Part print with two shaded views. Sizes in mm from the minimum x, y, z corner. A direction names the side the tool comes from. Round coordinates to 2 decimals unless told otherwise and drop trailing zeros. Order: outer loops, then holes, each group sorted by start corner. A loop starts at its lowest first (then second) coordinate and runs counter-clockwise, first axis right, second up. Notation, with made-up numbers: (38.25, 41.25) -> (82.25, 41.25) arc R18 cw to (82.25, 72.25) -> close; hole circle Ø11 at (74.5, 58). An arc over 180 degrees is marked (long way). Put each result on its own line as item: value. Start each with the question number.
Q1. Cut at A-A, the plane x = 62. List the corners of the cut face in (y, z) (3 decimals).
Q2. Cut at C-C, the plane z = 83.5. List the corners of the cut face in (x, y) (3 decimals).
Q3. Cut at D-D, the plane y = 91.5. List the corners of the cut face in (x, z) (3 decimals).
Q4. Probe L1, parallel to Z at x = 78, y = 137 (3 decimals); L2, parallel to X at y = 112, z = 59 (3 decimals); L3, parallel to Z at x = 91.5, y = 128. List the from-to ranges inside material, lowest first.
Q5. 3-axis set-ups, long thin cutter, end or side, ignore diameter. For the marked faces 5, 6, 7 and 8: which of +Z, -Z, +X, -X, +Y, -Y reach the whole face in a straight line?
Q6. Cut at B-B, the plane y = 141.5. List the corners of the cut face in (x, z) (3 decimals).
Q7. Flat gauge pins, fed straight in: P1, Ø4, axis at y = 65.5, z = 87.5, coming from the +X side; P2, Ø15, axis at y = 26, z = 79, coming from the +X side; P3, Ø15, axis at y = 82.5, z = 89, coming from the -X side; P4, Ø1.5, axis at x = 47.5, y = 135, coming from the -Z side. Where does each tip first touch, or does it go through?
Q8. Pull direction Z, two halves, no side cores. Call the marked faces 1, 2, 3 and 4: released by +Z, released by -Z, zero draft, split by the parting line, or undercut.
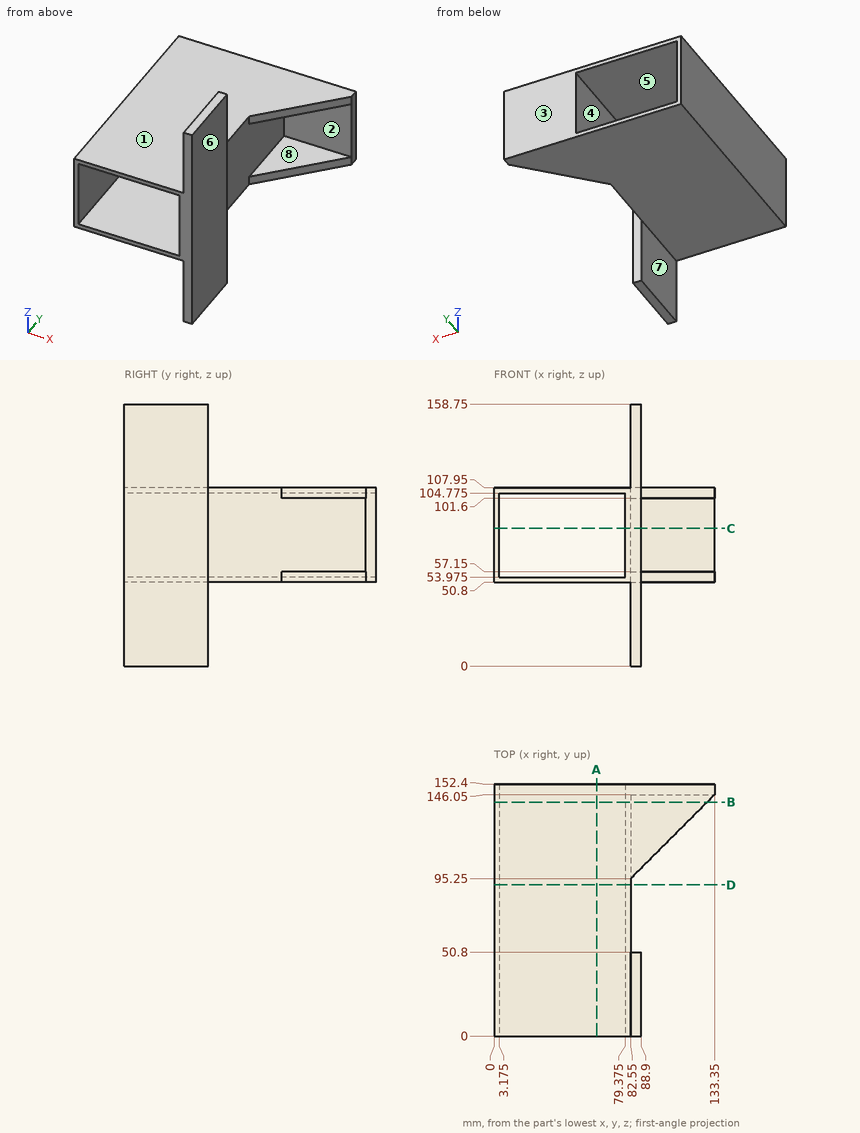
Ans:
1. outline: (0, 50.8) -> (152.4, 50.8) -> (152.4, 53.975) -> (0, 53.975) -> close; (0, 104.775) -> (152.4, 104.775) -> (152.4, 107.95) -> (0, 107.95) -> close
2. outline: (0, 0) -> (3.175, 0) -> (3.175, 152.4) -> (0, 152.4) -> close; (79.375, 0) -> (88.9, 0) -> (88.9, 50.8) -> (82.55, 50.8) -> (82.55, 146.05) -> (133.35, 146.05) -> (133.35, 152.4) -> (79.375, 152.4) -> close
3. outline: (0, 50.8) -> (82.55, 50.8) -> (82.55, 107.95) -> (0, 107.95) -> close; hole (3.175, 53.975) -> (79.375, 53.975) -> (79.375, 104.775) -> (3.175, 104.775) -> close
4. L1: z = 50.8 to 53.975, 104.775 to 107.95
4. L2: x = 0 to 3.175, 79.375 to 82.55
4. L3: z = 50.8 to 57.15, 101.6 to 107.95
5. face 5: +Y, -Y
5. face 6: +Z, -Z, +X, -Y
5. face 7: -Z, -X, +Y, -Y
5. face 8: +X
6. outline: (0, 50.8) -> (128.8, 50.8) -> (128.8, 57.15) -> (82.55, 57.15) -> (82.55, 101.6) -> (128.8, 101.6) -> (128.8, 107.95) -> (0, 107.95) -> close; hole (3.175, 53.975) -> (79.375, 53.975) -> (79.375, 104.775) -> (3.175, 104.775) -> close
7. P1: stops at x = 82.55
7. P2: stops at x = 88.9
7. P3: stops at x = 0
7. P4: stops at z = 50.8
8. face 1: released by +Z
8. face 2: undercut
8. face 3: zero draft
8. face 4: undercut
